Verification items for the finished model (mm, model axes). Face numbers are marked on the shaded views. A direction names the side the tool comes from. Round coordinates to 2 decimals unless told otherwise and drop trailing zeros. Write each loop counter-clockwise with the first axis right and the second up, starting at its lowest first coordinate (ties: lowest second). Pieces come first, ordered by that corner, then holes. Notation, with made-up numbers: M 7,-20 L 39,-20 A18 ccw 39,8 Z; hole C 62,34 d9. An arc over 180 degrees is marked long. One line per question, with ' | ' between items. Start each with the question number.
Q1. Cross-section at A-A (y = 10.5). Record the boundary of the cut face in (x, z), then the cut area to 3 significant figures.
Q2. Cross-section at B-B (z = 4.25). Record the boundary of the cut face in (x, y), then the cut area to 3 significant figures.
Q3. Cross-section at D-D (z = 8.25). Record the boundary of the cut face in (x, y).
Q4. Release check for a two-part mould opening along Y. For the marked faces 1, 2 and 3 record: released by +Y, released by -Y, zero draft, split by the parting line, or undercut.
Q5. Thickness scan on line 1 along Z through (x, y) = (3.25, 10.75); line 2 along X through (y, z) = (9, 1); line 3 along Y through (x, z) = (8, 7). Record the ranges inside material, lowest first. Write a range as from..to.
Q6. Cross-section at C-C (x = 8.5). Record the boundary of the cut face in (y, z), then the cut area to 3 significant figures.
Q7. Tool access check on the marked faces 4, 5 and 6. Record the directions out of +Z, -Z, +X, -X, +Y, -Y that give a thin tool (end or side, any length) a straight path to the whole face; none if there is none.
Q8. Gauge pin test, flat ends, axial feed: pin 1 (2 mm diameter, centred on x = 3, z = 8.5, fed in from +Y); pin 2 (4 mm diameter, centred on x = 7.5, z = 4.5, fed in from +Y); pin 3 (3 mm diameter, centred on y = 15.5, z = 5, fed in from -X); pin 4 (3 mm diameter, centred on y = 11.68, z = 5, fed in from +X). Record the tip position at first contact, or that the pin passes through.
from build123d import *

# Parameters (mm, degrees)
F1_DEPTH    = 10
F4_DEPTH    = 11.5542393178
F5_D        = 3.3
F6_T1_DEPTH = 27.5
F6_T3_DEPTH = 27.5
F6_T5_DEPTH = 21.0021683442


# Not quite as in the source:
# - a fillet or chamfer that OpenCascade refuses, or shapes differently, is made with other operations: its cross-section is extruded or revolved along the edge and cut away or added


with BuildPart() as f1:
    # F0 (on Top) → F1 (new body)
    with BuildSketch(Plane.XY):
        Polygon((4.0542393178, 8.6797312124), (4.0542393178, 18.6797312124), (1.5542393178, 18.6797312124), (1.5542393178, 8.6797312124), (1.5542393178, 6.1797312124), (11.5542393178, 6.1797312124), (11.5542393178, 8.6797312124), align=None)
    extrude(amount=F1_DEPTH)

    # F3 (on Right) → F4 (join, through all)
    with BuildSketch(Plane.YZ):
        Polygon((10.296677351, 17.1307598841), (6.1797312124, 10), (9.0664825583, 10), (13.183428697, 17.1307598841), align=None)
    extrude(amount=F4_DEPTH)

    # F5 (through all)
    with Locations(Plane.YZ.offset(4.0542393178)):
        with Locations((11.6797312124, 5)):
            Hole(F5_D / 2)

    # F6: fillet of radius 5 on 4 edges, made by hand

    # F6_s2 → F6_t1 (cut)
    with BuildSketch(Plane.YZ.offset(-10.9457606822)):
        with BuildLine():
            ThreePointArc((13.6797312124, 0), (17.2152651183, 1.4644660941), (18.6797312124, 5))
            Line((18.6797312124, 5), (18.6797312124, 0))
            Line((18.6797312124, 0), (13.6797312124, 0))
        make_face()
        with BuildLine():
            ThreePointArc((18.6797312124, 5), (17.2152651183, 8.5355339059), (13.6797312124, 10))
            Line((13.6797312124, 10), (18.6797312124, 10))
            Line((18.6797312124, 10), (18.6797312124, 5))
        make_face()
    extrude(amount=F6_T1_DEPTH, mode=Mode.SUBTRACT)

    # F6_s4 → F6_t3 (cut)
    with BuildSketch(Plane.XZ.offset(-21.1797312124)):
        with BuildLine():
            ThreePointArc((6.5542393178, 0), (10.0897732237, 1.4644660941), (11.5542393178, 5))
            Line((11.5542393178, 5), (11.5542393178, 0))
            Line((11.5542393178, 0), (6.5542393178, 0))
        make_face()
    extrude(amount=F6_T3_DEPTH, mode=Mode.SUBTRACT)

    # F6_s6 → F6_t5 (cut)
    with BuildSketch(Plane.XZ.offset(-18.1241910575)):
        with BuildLine():
            ThreePointArc((1.5542393178, 10), (0.4049590094, 11.6518912998), (0, 13.6230833997))
            Line((0, 13.6230833997), (0, 10))
            Line((0, 10), (1.5542393178, 10))
        make_face()
    extrude(amount=F6_T5_DEPTH, mode=Mode.SUBTRACT)


solid = f1.part
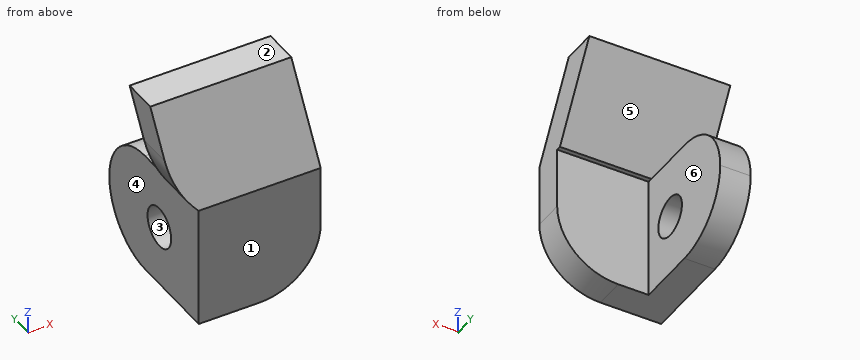
Determined:
1) outline: M 0,13.62 A5 ccw 0.13,12.48 L 11.55,12.48 L 11.55,17.13 L 0,17.13 Z; M 1.55,0 L 4.05,0 L 4.05,3.85 L 1.55,3.85 Z; M 1.55,6.15 L 4.05,6.15 L 4.05,10 L 1.55,10 Z | area: 72.9 mm²
2) outline: M 1.55,6.18 L 11.5,6.18 L 11.5,8.68 L 4.05,8.68 L 4.05,10.21 L 1.55,10.21 Z; M 1.55,13.15 L 4.05,13.15 L 4.05,18.62 L 1.55,18.62 Z | area: 42.4 mm²
3) outline: M 1.55,6.18 L 11.55,6.18 L 11.55,8.68 L 4.05,8.68 L 4.05,17.48 L 1.55,17.48 Z
4) face 1: released by -Y | face 2: zero draft | face 3: undercut
5) line 1: z = 0..3.64, 6.36..10, 12.92..17.13 | line 2: x = 1.55..4.05 | line 3: y = 6.18..8.68
6) outline: M 6.18,0.39 L 8.68,0.39 L 8.68,10 L 9.07,10 L 13.18,17.13 L 10.3,17.13 L 6.18,10 Z | area: 44.6 mm²
7) face 4: -Z, -X, +Y, -Y | face 5: +X, -X, +Y | face 6: -Z, +X, +Y
8) pin 1: stops at y = 18.01 | pin 2: stops at y = 8.68 | pin 3: stops at x = 1.55 | pin 4: passes through
